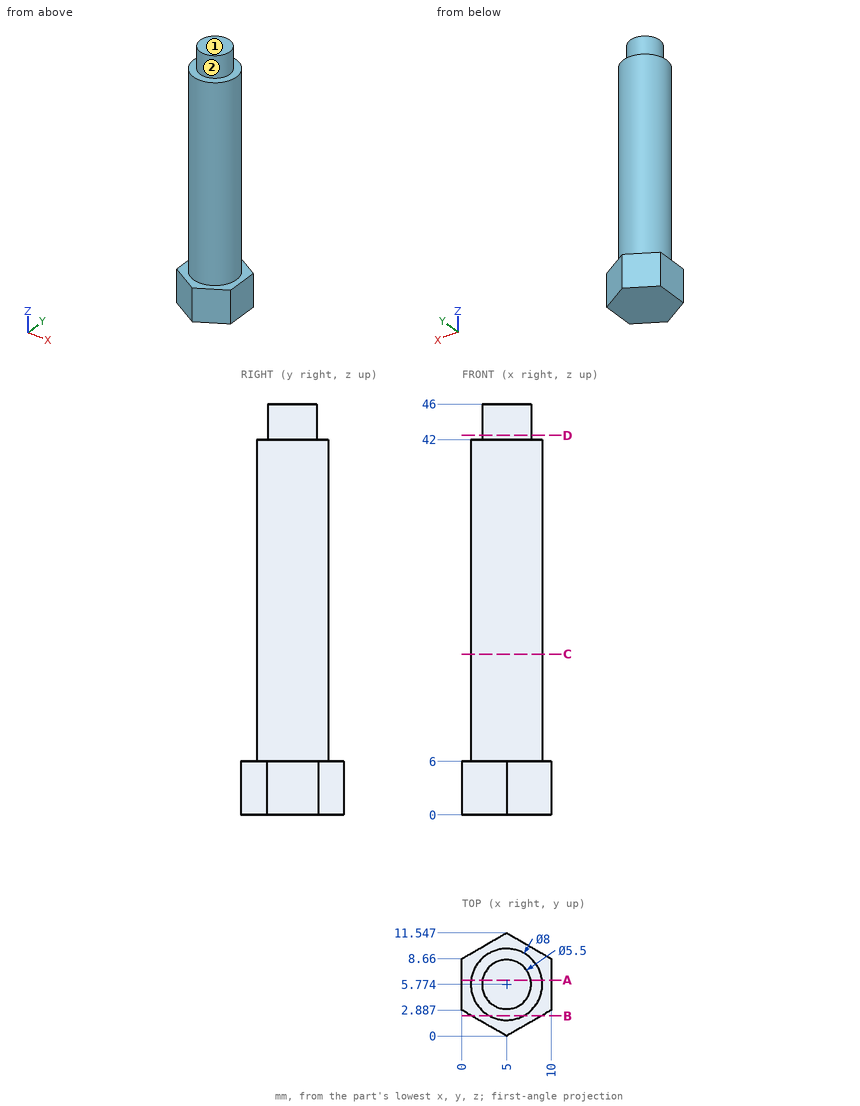
Print and shaded views of the part. All mm, measured from the part's lowest x, y and z. A direction names the side the tool comes from. Give positions to 0.01 mm unless a question says otherwise; leave off trailing zeros. Order: outer loops, then holes, each group sorted by start corner. A loop starts at its lowest first (then second) coordinate and runs counter-clockwise, first axis right, second up. Notation, with made-up numbers: M 29.25,11.25 L 75.25,11.25 A25 ccw 75.25,29.25 Z; hole C 11,85 d4. An arc over 180 degrees is marked long. Use one line per item in the form item = value.
Q1. Slice it at B-B, the plane y = 2.25. Write the cut outline in (x, z).
Conclusion:
outline = M 1.1,0 L 8.9,0 L 8.9,6 L 6.89,6 L 6.89,42 L 3.11,42 L 3.11,6 L 1.1,6 Z
Q2. Which spindle directions (+Z, -Z, +X, -X, +Y, -Y) get a long thin tool onto all of the face, cutting with end or side? Do the marked faces 1 and 2. Say none if no direction does.
Conclusion:
face_1 = +Z, +X, -X, +Y, -Y
face_2 = +Z
Q3. Slice it at D-D, the plane z = 42.5. Write the cut outline in (x, y).
Conclusion:
outline = C 5,5.77 d5.5
Q4. Slice it at C-C, the plane z = 18. Write the cut outline in (x, y).
Conclusion:
outline = C 5,5.77 d8
Q5. Slice it at A-A, the plane y = 6.25. Write the cut outline in (x, z), and give its area (3 significant figures).
Conclusion:
outline = M 0,0 L 10,0 L 10,6 L 8.97,6 L 8.97,42 L 7.71,42 L 7.71,46 L 2.29,46 L 2.29,42 L 1.03,42 L 1.03,6 L 0,6 Z
area = 368 mm2
Q6. Wall check: probe 1 along X at (y, z) = (5.5, 12); probe 2 along Y at (x, z) = (5.25, 29) (1 decimal); probe 3 along Z at (x, y) = (2, 4.5). Give the ranges that are in metal, low to high.
Conclusion:
probe_1 = 1.01 to 8.99
probe_2 = 1.8 to 9.8
probe_3 = 0 to 42
Q7. Pin check, flat tips, straight feed: P1, Ø4, axis at y = 8, z = 34, coming from the -X side; P2, Ø3, axis at x = 2, z = 27, coming from the -Y side (1 decimal); P3, Ø5, axis at x = 7, z = 25, coming from the -Y side. Stop position of each tip, or through.
Conclusion:
P1 = 1.01
P2 = 2.1
P3 = 1.77
